CAD build for the part. Positions are in the model's coordinates, mm. A direction names the side the tool comes from. Coordinates: 2 decimals unless noted, no trailing zeros. Order: outer loops, then holes, each group sorted by start corner. A loop starts at its lowest first (then second) coordinate and runs counter-clockwise, first axis right, second up. Notation, with made-up numbers: M 10,57 L 31,57 A11 cw 31,67 Z; hole C 16.25,-10.5 d1. An arc over 180 degrees is marked long. Write item = value, one per line.
Autodesk Fusion 360 part; units mm, degrees
sketch "base" plane through (0, 0, 0) normal (0, 0, 1) x (1, 0, 0)
  line L0 (-7.5707, -39.3146) -> (5.4293, -39.3146)
  line L1 (7.4293, -37.3146) -> (7.4293, -36.3146)
  line L2 (-8.5707, -35.3146) -> (-8.5707, -38.3146)
  line L3 (5.4293, -39.3146) -> (2.4293, -39.3146)
  line L4 (2.4293, -34.3146) -> (5.4293, -34.3146)
  line L5 (7.4293, -36.3146) -> (7.4293, -37.3146)
  line L6 (2.4293, -39.3146) -> (-2.5707, -39.3146)
  line L7 (-2.5707, -34.3146) -> (-2.5707, 33.4854)
  line L8 (-2.5707, 39.4854) -> (2.4293, 39.4854)
  line L9 (-7.5707, 39.4854) -> (5.4293, 39.4854)
  line L10 (7.4293, 37.4854) -> (7.4293, 35.4854)
  line L11 (-8.5707, 34.4854) -> (-8.5707, 38.4854)
  line L12 (2.4293, 33.4854) -> (2.4293, 23.1854) construction
  line L13 (2.4293, 23.1854) -> (5.4293, 23.1854)
  line L14 (7.4293, 21.1854) -> (7.4293, 19.1854)
  line L15 (5.4293, 17.1854) -> (4.4293, 17.1854)
  line L16 (2.4293, -34.3146) -> (2.4293, -24.0146) construction
  line L17 (2.4293, -24.0146) -> (5.4293, -24.0146)
  line L18 (7.4293, -22.0146) -> (7.4293, -21.0146)
  line L19 (5.4293, -19.0146) -> (4.4293, -19.0146)
  line L20 (2.4293, -24.0146) -> (2.4293, -34.3146)
  line L21 (5.4293, -34.3146) -> (2.4293, -34.3146)
  line L22 (-2.5707, -34.3146) -> (-7.5707, -34.3146)
  line L23 (2.4293, 33.4854) -> (2.4293, 23.1854)
  line L24 (2.4293, 15.1854) -> (2.4293, -17.0146)
  line L25 (5.4293, 33.4854) -> (2.4293, 33.4854)
  line L26 (-2.5707, 33.4854) -> (-7.5707, 33.4854)
  arc A0 (-7.5707, 39.4854) -> (-8.5707, 38.4854) centre (-7.5707, 38.4854) ccw
  arc A1 (-8.5707, 34.4854) -> (-7.5707, 33.4854) centre (-7.5707, 34.4854) ccw
  arc A2 (-7.5707, -34.3146) -> (-8.5707, -35.3146) centre (-7.5707, -35.3146) ccw
  arc A3 (-8.5707, -38.3146) -> (-7.5707, -39.3146) centre (-7.5707, -38.3146) ccw
  arc A4 (7.4293, 37.4854) -> (5.4293, 39.4854) centre (5.4293, 37.4854) ccw
  arc A5 (5.4293, 33.4854) -> (7.4293, 35.4854) centre (5.4293, 35.4854) ccw
  arc A6 (7.4293, 21.1854) -> (5.4293, 23.1854) centre (5.4293, 21.1854) ccw
  arc A7 (5.4293, 17.1854) -> (7.4293, 19.1854) centre (5.4293, 19.1854) ccw
  arc A8 (4.4293, 17.1854) -> (2.4293, 15.1854) centre (4.4293, 15.1854) ccw
  arc A9 (2.4293, -17.0146) -> (4.4293, -19.0146) centre (4.4293, -17.0146) ccw
  arc A10 (7.4293, -21.0146) -> (5.4293, -19.0146) centre (5.4293, -21.0146) ccw
  arc A11 (5.4293, -24.0146) -> (7.4293, -22.0146) centre (5.4293, -22.0146) ccw
  arc A12 (7.4293, -36.3146) -> (5.4293, -34.3146) centre (5.4293, -36.3146) ccw
  arc A13 (5.4293, -39.3146) -> (7.4293, -37.3146) centre (5.4293, -37.3146) ccw
  point P0 (-8.5707, -39.3146)
  point P1 (-8.5707, -34.3146)
  point P2 (-8.5707, 39.4854)
  point P3 (7.4293, 39.4854)
  point P4 (-8.5707, 33.4854)
  point P5 (7.4293, 23.1854)
  point P6 (2.4293, 17.1854)
  point P7 (7.4293, -24.0146)
  point P8 (2.4293, -19.0146)
  dimension "d2" = 5
  dimension "d4" = 5
  dimension "d5" = 78.8
  dimension "d6" = 16
  dimension "d7" = 6
  dimension "d8" = 6
  dimension "d9" = 10.3
  dimension "d10" = 5
  dimension "d11" = 6
  dimension "d12" = 10.3
  dimension "d13" = 5
  dimension "d14" = 5
  dimension "d15" = 1
  dimension "d16" = 2
  dimension "d17" = 2
extrude "Extrude1" add sketch "base" along normal blind 30
sketch "right-holes" plane through (2.4293, 0, 0) normal (1, 0, 0) x (0, 1, 0)
  line L0 (23.1854, 0) -> (33.4854, 0)
  line L1 (33.4854, 0) -> (33.4854, 30)
  line L2 (33.4854, 30) -> (23.1854, 30)
  line L3 (23.1854, 30) -> (23.1854, 0)
  line L4 (33.4854, 30) -> (28.3354, 30)
  line L5 (33.4854, 22.5) -> (33.4854, 30)
  circle A0 centre (28.3354, 22.5) radius 2.25
  line L6 (28.3354, 30) -> (28.3354, 15) construction
  line L7 (23.1854, 15) -> (33.4854, 15) construction
  circle A1 centre (28.3354, 7.5) radius 2.25
  dimension "d20" = 5.15
  dimension "d21" = 7.5
  dimension "d22" = 4.5
  dimension "d23" = 15
  dimension "d24" = 7.5
sketch "left-holes" plane through (2.4293, 0, 0) normal (1, 0, 0) x (0, 1, 0)
  line L0 (-34.3146, 0) -> (-24.0146, 0)
  line L1 (-24.0146, 0) -> (-24.0146, 30)
  line L2 (-24.0146, 30) -> (-34.3146, 30)
  line L3 (-34.3146, 30) -> (-34.3146, 0)
  line L4 (-34.3146, 30) -> (-29.1646, 30)
  line L5 (-29.1646, 30) -> (-29.1646, 22.5) construction
  line L6 (-29.1646, 22.5) -> (-34.3146, 22.5) construction
  line L7 (-34.3146, 22.5) -> (-34.3146, 30)
  circle A0 centre (-29.1646, 22.5) radius 2.25
  line L8 (-24.0146, 15) -> (-34.3146, 15) construction
  circle A1 centre (-29.1646, 7.5) radius 2.25
  dimension "d25" = 5.15
  dimension "d26" = 4.5
extrude "Extrude2" cut sketch "left-holes" sketch "right-holes" against normal blind 16 contours A0 | A1 of sketch 2 contours A0 | A1
fillet "Fillet1" radius 1 62 edges at (-5.0707, -34.3146, 30) (-8.2778, -34.6075, 30) (-8.5707, -36.8146, 30) (-8.2778, -39.0217, 30) (-1.0707, -39.3146, 30) (6.8435, -38.7288, 30) (7.4293, -36.8146, 30) (6.8435, -34.9004, 30) (3.9293, -34.3146, 30) (-5.0707, -34.3146, 0) (-8.2778, -34.6075, 0) (-8.5707, -36.8146, 0) (-8.2778, -39.0217, 0) (-1.0707, -39.3146, 0) (6.8435, -38.7288, 0) (7.4293, -36.8146, 0) (6.8435, -34.9004, 0) (3.9293, -34.3146, 0) (3.9293, -24.0146, 0) (6.8435, -23.4288, 0) (7.4293, -21.5146, 0) (6.8435, -19.6004, 0) (4.9293, -19.0146, 0) (3.0151, -18.4288, 0) (2.4293, -0.9146, 0) (3.0151, 16.5996, 0) (4.9293, 17.1854, 0) (6.8435, 17.7712, 0) (7.4293, 20.1854, 0) (6.8435, 22.5996, 0) (3.9293, 23.1854, 0) (3.9293, -24.0146, 30) (6.8435, -23.4288, 30) (7.4293, -21.5146, 30) (6.8435, -19.6004, 30) (4.9293, -19.0146, 30) (3.0151, -18.4288, 30) (2.4293, -0.9146, 30) (3.0151, 16.5996, 30) (4.9293, 17.1854, 30) (6.8435, 17.7712, 30) (7.4293, 20.1854, 30) (6.8435, 22.5996, 30) (3.9293, 23.1854, 30) (3.9293, 33.4854, 30) (6.8435, 34.0712, 30) (7.4293, 36.4854, 30) (6.8435, 38.8996, 30) (-1.0707, 39.4854, 30) (-8.2778, 39.1925, 30) (-8.5707, 36.4854, 30) (-8.2778, 33.7783, 30) (-5.0707, 33.4854, 30) (-5.0707, 33.4854, 0) (-8.2778, 33.7783, 0) (-8.5707, 36.4854, 0) (-8.2778, 39.1925, 0) (-1.0707, 39.4854, 0) (6.8435, 38.8996, 0) (7.4293, 36.4854, 0) (6.8435, 34.0712, 0) (3.9293, 33.4854, 0)
(1) Slice it at C-C, the plane x = -0.25. Write the cut outline in (y, z), then the cut area to 3 significant figures.
Evaluation:
outline = M -39.31,1 A1 ccw -38.31,0 L 38.49,0 A1 ccw 39.49,1 L 39.49,29 A1 ccw 38.49,30 L -38.31,30 A1 ccw -39.31,29 Z; hole C -29.16,7.5 d4.5; hole C -29.16,22.5 d4.5; hole C 28.34,7.5 d4.5; hole C 28.34,22.5 d4.5
area = 2,300 mm²
(2) Pin check, flat tips, straight feed: pin 1 Ø2 at (y, z) = (-27, 22.5) entering from +X; pin 2 Ø3.5 at (y, z) = (-29.16, 7.5) entering from -X; pin 3 Ø13.5 at (y, z) = (-29, 8) entering from +X; pin 4 Ø10 at (y, z) = (27, 8.5) entering from +X. Stop position of each tip, or through.
Evaluation:
pin_1 = 2.43
pin_2 = through
pin_3 = 7.42
pin_4 = 7.26
(3) Slice it at A-A, the plane x = -5.25. Write the cut outline in (y, z).
Evaluation:
outline = M -39.31,1 A1 ccw -38.31,0 L -35.31,0 A1 ccw -34.31,1 L -34.31,29 A1 ccw -35.31,30 L -38.31,30 A1 ccw -39.31,29 Z; M 33.49,1 A1 ccw 34.49,0 L 38.49,0 A1 ccw 39.49,1 L 39.49,29 A1 ccw 38.49,30 L 34.49,30 A1 ccw 33.49,29 Z
(4) Wall check: line 1 (Y direction, x = 4.5, z = 25); line 2 (Y direction, x = -4.5, z = 4); line 3 (Y direction, x = -1.5, z = 23). Give the ranges that are in metal, low to high. Write a range as from..to.
Evaluation:
line_1 = -39.31..-34.31, -24.01..-19.01, 17.19..23.19, 33.49..39.49
line_2 = -39.31..-34.31, 33.49..39.49
line_3 = -39.31..-31.36, -26.97..26.14, 30.53..39.49
(5) Slice it at D-D, the plane z = 7.5. State how many separate pieces and enclosed holes the cut face has, then the cut area to 3 significant figures.
Evaluation:
separate_pieces = 3
enclosed_holes = 0
area = 519 mm²
(6) Tool access for faces 1 (the face through (4, -24.015, 15)), 2 (the face through (-5, 33.485, 15)), 3 (the face through (-1, 39.485, 15)): list every direction of +Z, -Z, +X, -X, +Y, -Y with a clear straight run to the whole face (end or side of a thin tool).
Evaluation:
face_1 = +Z, -Z, +X
face_2 = +Z, -Z, -X
face_3 = +Z, -Z, +X, -X, +Y
(7) Pull direction Z, two halves, no side cores. Call faces 4 (the face through (6.86, 34.09, 14.8)), 5 (the face through (-0.04, 26.55, 21.13)), 6 (the face through (-1, 9, 0)): +Z half, -Z half, draft (parallel to the pull), parting line (faces both ways), or undercut.
Evaluation:
face_4 = draft
face_5 = undercut
face_6 = -Z half
